Here's the drawing with two shaded views (mm, measured from the low corner). I have some questions. A direction names the side the tool comes from. Coordinates: 2 decimals unless noted, no trailing zeros. Loops run counter-clockwise (first coordinate to the right, second up) from the corner with the lowest first, then second, coordinate; pieces in that order, holes last. Notation, with made-up numbers: M 87,-19.75 L 131,-19.75 A30 ccw 131,19.25 Z; hole C 38.5,-10 d3. An arc over 180 degrees is marked long. Use one line per item in the form item = value. Start each with the question number.
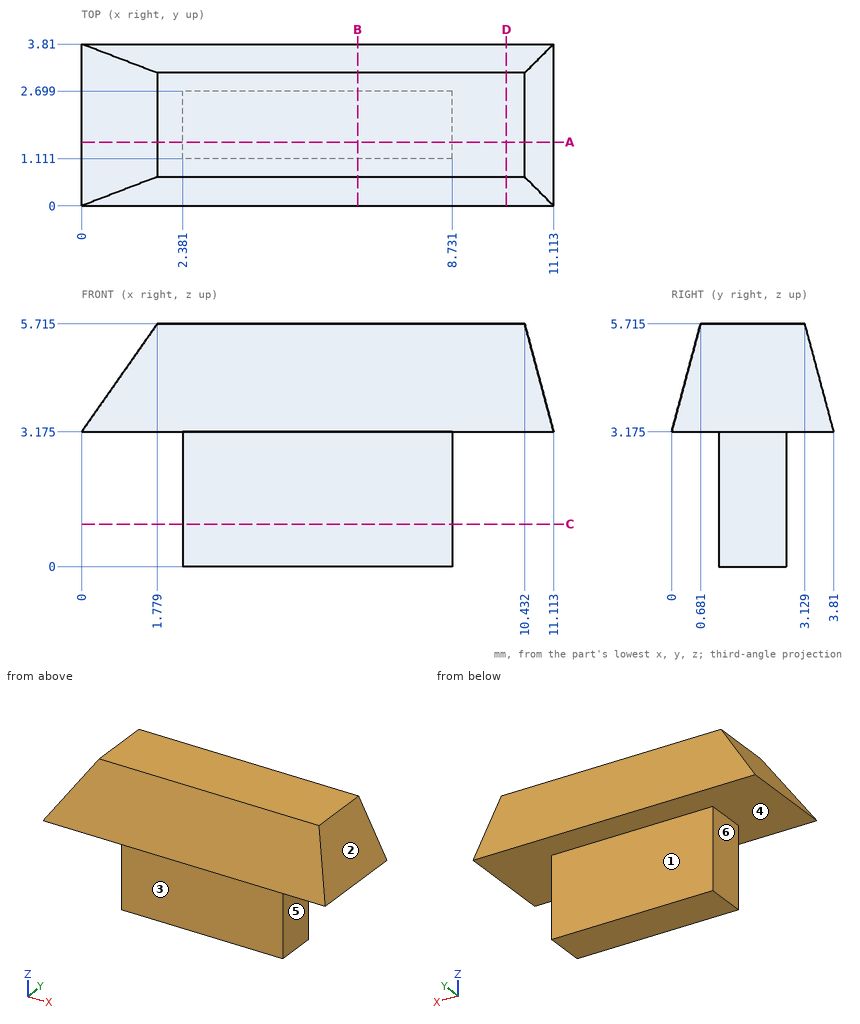
Item 1: For the marked faces 1, 2 and 3, which set-ups out of +Z, -Z, +X, -X, +Y, -Y let a thin tool reach every point of the face, with its end or its side?
Item 2: I'm going to push flat-ended pins straight in: P1, Ø2, axis at x = 1.5, z = 2, coming from the +Y side; P2, Ø0.8, axis at y = 1.5, z = 2, coming from the -X side; P3, Ø0.5, axis at y = 1.5, z = 2, coming from the +X side. Where does each tip first touch, or does it pass through?
Item 3: Please list where these lines run through material, in increasing order: line 1 along X through (y, z) = (2.45, 1.45); line 2 along Y through (x, z) = (3.5, 2.1); line 3 along Z through (x, y) = (9.75, 3) (1 decimal).
Item 4: I want a section at C-C (z = 1). Write out the boundary of the cut face in (x, y), plus the area to 3 significant figures.
Item 5: I want a section at A-A (y = 1.5). Write out the boundary of the cut face in (x, z) (1 decimal).
Item 6: I want a section at D-D (x = 10). Write out the boundary of the cut face in (y, z) (1 decimal).
Item 7: Thinking about a two-plate mould opening in X: for the marked faces 4, 5 and 6, which applies, pulls with the +X half, pulls with the -X half, needs draft (parallel to the pull), parting line crosses it, or undercut?
Item 8: I want a section at B-B (x = 6.5). Write out the boundary of the cut face in (y, z) (1 decimal), plus the area to 3 significant figures.
Worked answers:
q1.face_1 = -Z, +X, -X, +Y
q1.face_2 = +Z, +X, +Y, -Y
q1.face_3 = -Z, +X, -X, -Y
q2.P1 = 2.7
q2.P2 = 2.38
q2.P3 = 8.73
q3.line_1 = 2.38 to 8.73
q3.line_2 = 1.11 to 2.7
q3.line_3 = 3.2 to 5.7
q4.outline = M 2.38,1.11 L 8.73,1.11 L 8.73,2.7 L 2.38,2.7 Z
q4.area = 10.1 mm²
q5.outline = M 0,3.2 L 2.4,3.2 L 2.4,0 L 8.7,0 L 8.7,3.2 L 11.1,3.2 L 10.4,5.7 L 1.8,5.7 Z
q6.outline = M 0,3.2 L 3.8,3.2 L 3.1,5.7 L 0.7,5.7 Z
q7.face_4 = needs draft
q7.face_5 = pulls with the +X half
q7.face_6 = pulls with the -X half
q8.outline = M 0,3.2 L 1.1,3.2 L 1.1,0 L 2.7,0 L 2.7,3.2 L 3.8,3.2 L 3.1,5.7 L 0.7,5.7 Z
q8.area = 13.0 mm²
